Geometry: final body of the model. Coordinates: model frame, mm. A direction names the side the tool comes from. Round coordinates to 2 decimals unless told otherwise and drop trailing zeros. One line per item, written item: value. Start each with the question number.
Autodesk Fusion 360 part; units mm, degrees
sketch "Sketch1" plane through (0, 0, 0) normal (0, 0, 1) x (1, 0, 0)
  circle A0 centre (0, 0) radius 14
  dimension "d1" = 28
extrude "Extrude1" add sketch "Sketch1" along normal blind 3 draft -23
sketch "Sketch2" plane through (0, 0, 3) normal (0, 0, 1) x (-1, 0, 0)
  circle A0 centre (0, 0) radius 12.7266
sketch "Sketch3" plane through (0, 0, 3) normal (0, 0, 1) x (-1, 0, 0)
sketch "Sketch4" plane through (0, 0, 3) normal (0, 0, 1) x (-1, 0, 0)
  circle A0 centre (0, 0) radius 10.625
  dimension "d5" = 21.25
extrude "Extrude2" add sketch "Sketch4" along normal blind 15
sketch "Sketch5" plane through (0, 0, 18) normal (0, 0, 1) x (-1, 0, 0)
  circle A0 centre (0, 0) radius 10.625
  line L0 (3.3198, -5.75) -> (6.6395, 0)
  line L1 (6.6395, 0) -> (3.3198, 5.75)
  line L2 (3.3198, 5.75) -> (-3.3198, 5.75)
  line L3 (-3.3198, 5.75) -> (-6.6395, 0)
  line L4 (-6.6395, 0) -> (-3.3198, -5.75)
  line L5 (-3.3198, -5.75) -> (3.3198, -5.75)
  dimension "d8" = 5.75
extrude "Extrude3" cut sketch "Sketch5" against normal blind 15 contours L0 L1 L2 L3 L4 L5
hole "Hole1" at (-0.0502, 0.0031, 0) direction (0, 0, 1) diameter 7 depth 3 tip angle 180
sketch "1/4\" Bolt Hole" plane through (0, 0, 0) normal (0, 0, -1) x (1, 0, 0)
  circle A0 centre (-0.0502, -0.0031) radius 3.5
  circle A1 centre (0, 0) radius 14
sketch "Sketch7" plane through (0, 0, 18) normal (0, 0, 1) x (-1, 0, 0)
sketch "Sketch8" plane through (0, 0, 18) normal (0, 0, 1) x (-1, 0, 0)
(1) Line query: probe 1 along X at (y, z) = (3.75, 9.25); probe 2 along Y at (x, z) = (-1, 13.75); probe 3 along Z at (x, y) = (9.5, -7.25). Output: solid intervals per line, ascending.
(2) Set-up query: faces 1 (the face through (-4.956, 2.915, 10.605)), 2 (the face through (-5, 5, 18)). Return all of +Z, -Z, +X, -X, +Y, -Y with unobstructed straight access to the full face (end or side cutting, diameter ignored); none if empty.
(3) Pull-direction query (X, two-part tool) for faces 3 (the face through (3, -3, 0)), 4 (the face through (-3, -3, 3)), 5 (the face through (-5.003, -2.835, 10.605)), 6 (the face through (-2.8, 12.5, 2.8)); classes: pulls with the +X half, pulls with the -X half, needs draft (parallel to the pull), parting line crosses it, or undercut.
(4) Pin query (flat end, axial travel): pin 1 (3 mm diameter, centred on y = -3, z = 15.5, fed in from +X); pin 2 (6 mm diameter, centred on x = 2, y = 0.5, fed in from +Z); pin 3 (2 mm diameter, centred on x = 1, z = 9, fed in from +Y) (3 decimals). Return the tip coordinate at first contact, or that it passes through.
Results list:
1. probe 1: x = -9.94 to -4.47, 4.47 to 9.94
1. probe 2: y = -10.58 to -5.75, 5.75 to 10.58
1. probe 3: z = 0 to 3
2. face 1: +Z
2. face 2: +Z, +X, -X, +Y, -Y
3. face 3: needs draft
3. face 4: undercut
3. face 5: undercut
3. face 6: parting line crosses it
4. pin 1: stops at x = 10.52
4. pin 2: stops at z = 3
4. pin 3: stops at y = 10.625
